from build123d import *

# Parameters (mm, degrees)
BOSS_EXTRUDE4_DEPTH = 107
BOSS_EXTRUDE5_DEPTH = 2.31
SKETCH7_W           = 102.38
SKETCH7_H           = 83.08
CUT_EXTRUDE4_DEPTH  = 2.31
BOSS_EXTRUDE6_DEPTH = 2.31
CUT_EXTRUDE6_DEPTH  = 2.31
CUT_EXTRUDE7_DEPTH  = 70
SKETCH12_W          = 91.85
SKETCH12_H          = 11.6
CUT_EXTRUDE8_DEPTH  = 90


with BuildPart() as part:
    # Sketch1 → Boss-Extrude4 (new body)
    with BuildSketch(Plane(origin=(0, 0, 0), x_dir=(0, 0, -1), z_dir=(1, 0, 0))):
        with BuildLine():
            Line((0, 0), (87.7, 0))
            Line((87.7, 0), (87.7, 14.19))
            ThreePointArc((87.7, 14.19), (87.023416665, 15.823416665), (85.39, 16.5))
            Line((85.39, 16.5), (76.167, 16.5))
            ThreePointArc((76.167, 16.5), (74.533583335, 17.176583335), (73.857, 18.81))
            Line((73.857, 18.81), (73.857, 34.19))
            ThreePointArc((73.857, 34.19), (73.180416665, 35.823416665), (71.547, 36.5))
            Line((71.547, 36.5), (69.1628, 36.5))
            ThreePointArc((69.1628, 36.5), (67.529383335, 37.176583335), (66.8528, 38.81))
            Line((66.8528, 38.81), (66.8528, 45.417647019))
            ThreePointArc((66.8528, 45.417647019), (43.8531, 48.5), (20.8534, 45.417647019))
            Line((20.8534, 45.417647019), (20.8534, 38.81))
            ThreePointArc((20.8534, 38.81), (20.176816665, 37.176583335), (18.5434, 36.5))
            Line((18.5434, 36.5), (16.153, 36.5))
            ThreePointArc((16.153, 36.5), (14.519583335, 35.823416665), (13.843, 34.19))
            Line((13.843, 34.19), (13.843, 18.81))
            ThreePointArc((13.843, 18.81), (13.166416665, 17.176583335), (11.533, 16.5))
            Line((11.533, 16.5), (2.31, 16.5))
            ThreePointArc((2.31, 16.5), (0.676583335, 15.823416665), (0, 14.19))
            Line((0, 14.19), (0, 0))
        make_face()
        with BuildLine():
            Line((16.153, 34.19), (16.153, 18.81))
            ThreePointArc((16.153, 18.81), (14.799833329, 15.543166671), (11.533, 14.19))
            Line((11.533, 14.19), (2.31, 14.19))
            Line((2.31, 14.19), (2.31, 2.31))
            Line((2.31, 2.31), (85.39, 2.31))
            Line((85.39, 2.31), (85.39, 14.19))
            Line((85.39, 14.19), (76.167, 14.19))
            ThreePointArc((76.167, 14.19), (72.900166671, 15.543166671), (71.547, 18.81))
            Line((71.547, 18.81), (71.547, 34.19))
            Line((71.547, 34.19), (69.1628, 34.19))
            ThreePointArc((69.1628, 34.19), (65.895966671, 35.543166671), (64.5428, 38.81))
            Line((64.5428, 38.81), (64.5428, 43.634774003))
            ThreePointArc((64.5428, 43.634774003), (43.8531, 46.19), (23.1634, 43.634774003))
            Line((23.1634, 43.634774003), (23.1634, 38.81))
            ThreePointArc((23.1634, 38.81), (21.810233329, 35.543166671), (18.5434, 34.19))
            Line((18.5434, 34.19), (16.153, 34.19))
        make_face(mode=Mode.SUBTRACT)
    extrude(amount=BOSS_EXTRUDE4_DEPTH)

    # Sketch6 → Boss-Extrude5 (add)
    with BuildSketch(Plane.ZY):
        with BuildLine():
            Line((-85.39, 14.19), (-85.39, 2.31))
            Line((-85.39, 2.31), (-2.31, 2.31))
            Line((-2.31, 2.31), (-2.31, 14.19))
            Line((-2.31, 14.19), (-11.533, 14.19))
            ThreePointArc((-11.533, 14.19), (-14.799833329, 15.543166671), (-16.153, 18.81))
            Line((-16.153, 18.81), (-16.153, 34.19))
            Line((-16.153, 34.19), (-18.5434, 34.19))
            ThreePointArc((-18.5434, 34.19), (-21.810233329, 35.543166671), (-23.1634, 38.81))
            Line((-23.1634, 38.81), (-23.1634, 43.634774003))
            ThreePointArc((-23.1634, 43.634774003), (-43.8531, 46.19), (-64.5428, 43.634774003))
            Line((-64.5428, 43.634774003), (-64.5428, 38.81))
            ThreePointArc((-64.5428, 38.81), (-65.895966671, 35.543166671), (-69.1628, 34.19))
            ThreePointArc((-69.1628, 34.19), (-69.258906021, 34.189020865), (-69.355012042, 34.19))
            Line((-69.355012042, 34.19), (-71.547, 34.19))
            Line((-71.547, 34.19), (-71.547, 18.81))
            ThreePointArc((-71.547, 18.81), (-72.900166671, 15.543166671), (-76.167, 14.19))
            Line((-76.167, 14.19), (-85.39, 14.19))
        make_face()
    extrude(amount=-BOSS_EXTRUDE5_DEPTH)

    # Sketch7 → Cut-Extrude4 (cut)
    with BuildSketch(Plane.XZ):
        with Locations((53.5, -43.85)):
            Rectangle(SKETCH7_W, SKETCH7_H)
    extrude(amount=-CUT_EXTRUDE4_DEPTH, mode=Mode.SUBTRACT)

    # Sketch8 → Boss-Extrude6 (add)
    with BuildSketch(Plane(origin=(107, 0, 0), x_dir=(0, 0, -1), z_dir=(1, 0, 0))):
        with BuildLine():
            Line((2.31, 14.19), (2.31, 2.31))
            Line((2.31, 2.31), (85.39, 2.31))
            Line((85.39, 2.31), (85.39, 14.19))
            Line((85.39, 14.19), (76.167, 14.19))
            ThreePointArc((76.167, 14.19), (72.900166671, 15.543166671), (71.547, 18.81))
            Line((71.547, 18.81), (71.547, 34.19))
            Line((71.547, 34.19), (69.355012042, 34.19))
            ThreePointArc((69.355012042, 34.19), (69.258906021, 34.189020865), (69.1628, 34.19))
            ThreePointArc((69.1628, 34.19), (65.895966671, 35.543166671), (64.5428, 38.81))
            Line((64.5428, 38.81), (64.5428, 43.634774003))
            ThreePointArc((64.5428, 43.634774003), (43.8531, 46.19), (23.1634, 43.634774003))
            Line((23.1634, 43.634774003), (23.1634, 38.81))
            ThreePointArc((23.1634, 38.81), (21.810233329, 35.543166671), (18.5434, 34.19))
            Line((18.5434, 34.19), (16.153, 34.19))
            Line((16.153, 34.19), (16.153, 18.81))
            ThreePointArc((16.153, 18.81), (14.799833329, 15.543166671), (11.533, 14.19))
            Line((11.533, 14.19), (2.31, 14.19))
        make_face()
    extrude(amount=-BOSS_EXTRUDE6_DEPTH)

    # Sketch9 → Cut-Extrude6 (cut)
    with BuildSketch(Plane(origin=(0, 16.5, 0), x_dir=(1, 0, 0), z_dir=(0, 1, 0))):
        with BuildLine():
            Line((25, 83.7785), (82, 83.7785))
            ThreePointArc((82, 83.7785), (85, 80.7785), (82, 77.7785))
            Line((82, 77.7785), (25, 77.7785))
            ThreePointArc((25, 77.7785), (22, 80.7785), (25, 83.7785))
        make_face()
        with BuildLine():
            Line((25, 9.9215), (82, 9.9215))
            ThreePointArc((82, 9.9215), (85, 6.9215), (82, 3.9215))
            Line((82, 3.9215), (25, 3.9215))
            ThreePointArc((25, 3.9215), (22, 6.9215), (25, 9.9215))
        make_face()
    extrude(amount=-CUT_EXTRUDE6_DEPTH, mode=Mode.SUBTRACT)

    # Sketch11 → Cut-Extrude7 (cut)
    with BuildSketch(Plane.XY.offset(-13.843)):
        with BuildLine():
            Line((28.648320597, 30.5), (28.648320597, 22.5))
            ThreePointArc((28.648320597, 22.5), (29.898320597, 21.25), (31.148320597, 22.5))
            Line((31.148320597, 22.5), (31.148320597, 30.5))
            ThreePointArc((31.148320597, 30.5), (29.898320597, 31.75), (28.648320597, 30.5))
        make_face()
        with BuildLine():
            Line((38.648320597, 30.5), (38.648320597, 22.5))
            ThreePointArc((38.648320597, 22.5), (39.898320597, 21.25), (41.148320597, 22.5))
            Line((41.148320597, 22.5), (41.148320597, 30.5))
            ThreePointArc((41.148320597, 30.5), (39.898320597, 31.75), (38.648320597, 30.5))
        make_face()
        with BuildLine():
            Line((43.648320597, 30.5), (43.648320597, 22.5))
            ThreePointArc((43.648320597, 22.5), (44.898320597, 21.25), (46.148320597, 22.5))
            Line((46.148320597, 22.5), (46.148320597, 30.5))
            ThreePointArc((46.148320597, 30.5), (44.898320597, 31.75), (43.648320597, 30.5))
        make_face()
        with BuildLine():
            Line((48.648320597, 30.5), (48.648320597, 22.5))
            ThreePointArc((48.648320597, 22.5), (49.898320597, 21.25), (51.148320597, 22.5))
            Line((51.148320597, 22.5), (51.148320597, 30.5))
            ThreePointArc((51.148320597, 30.5), (49.898320597, 31.75), (48.648320597, 30.5))
        make_face()
        with BuildLine():
            Line((58.648320597, 30.5), (58.648320597, 22.5))
            ThreePointArc((58.648320597, 22.5), (59.898320597, 21.25), (61.148320597, 22.5))
            Line((61.148320597, 22.5), (61.148320597, 30.5))
            ThreePointArc((61.148320597, 30.5), (59.898320597, 31.75), (58.648320597, 30.5))
        make_face()
        with BuildLine():
            Line((63.648320597, 30.5), (63.648320597, 22.5))
            ThreePointArc((63.648320597, 22.5), (64.898320597, 21.25), (66.148320597, 22.5))
            Line((66.148320597, 22.5), (66.148320597, 30.5))
            ThreePointArc((66.148320597, 30.5), (64.898320597, 31.75), (63.648320597, 30.5))
        make_face()
        with BuildLine():
            Line((33.648320597, 30.5), (33.648320597, 22.5))
            ThreePointArc((33.648320597, 22.5), (34.898320597, 21.25), (36.148320597, 22.5))
            Line((36.148320597, 22.5), (36.148320597, 30.5))
            ThreePointArc((36.148320597, 30.5), (34.898320597, 31.75), (33.648320597, 30.5))
        make_face()
        with BuildLine():
            Line((53.648320597, 30.5), (53.648320597, 22.5))
            ThreePointArc((53.648320597, 22.5), (54.898320597, 21.25), (56.148320597, 22.5))
            Line((56.148320597, 22.5), (56.148320597, 30.5))
            ThreePointArc((56.148320597, 30.5), (54.898320597, 31.75), (53.648320597, 30.5))
        make_face()
        with BuildLine():
            Line((68.648320597, 30.5), (68.648320597, 22.5))
            ThreePointArc((68.648320597, 22.5), (69.898320597, 21.25), (71.148320597, 22.5))
            Line((71.148320597, 22.5), (71.148320597, 30.5))
            ThreePointArc((71.148320597, 30.5), (69.898320597, 31.75), (68.648320597, 30.5))
        make_face()
        with BuildLine():
            Line((76.148320597, 30.5), (76.148320597, 22.5))
            ThreePointArc((76.148320597, 22.5), (74.898320597, 21.25), (73.648320597, 22.5))
            Line((73.648320597, 22.5), (73.648320597, 30.5))
            ThreePointArc((73.648320597, 30.5), (74.898320597, 31.75), (76.148320597, 30.5))
        make_face()
        with BuildLine():
            Line((78.648320597, 30.5), (78.648320597, 22.5))
            ThreePointArc((78.648320597, 22.5), (79.898320597, 21.25), (81.148320597, 22.5))
            Line((81.148320597, 22.5), (81.148320597, 30.5))
            ThreePointArc((81.148320597, 30.5), (79.898320597, 31.75), (78.648320597, 30.5))
        make_face()
    extrude(amount=-CUT_EXTRUDE7_DEPTH, mode=Mode.SUBTRACT)

    # Sketch12 → Cut-Extrude8 (cut)
    with BuildSketch(Plane.XY):
        with Locations((53.505, 5.8)):
            Rectangle(SKETCH12_W, SKETCH12_H)
    extrude(amount=-CUT_EXTRUDE8_DEPTH, mode=Mode.SUBTRACT)


solid = part.part
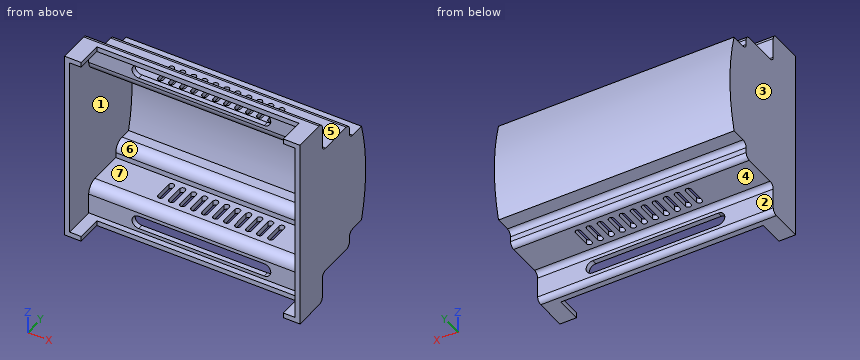
Can you work these out from the model? Positions are in its coordinate system, mm. Face numbers are marked on the shaded views. A direction names the side the tool comes from. Coordinates: 2 decimals unless noted, no trailing zeros. Loops run counter-clockwise (first coordinate to the right, second up) from the corner with the lowest first, then second, coordinate; pieces in that order, holes last. Notation, with made-up numbers: M 19.25,-28.5 L 28.25,-28.5 A17 cw 28.25,4.5 Z; hole C 89.25,-12.5 d8. An arc over 180 degrees is marked long. Return JSON: item names as keys, results as strings. Group by question number.
Item 1: Thinking about a two-plate mould opening in Z: for the marked faces 4, 5, 6 and 7, which applies, released by +Z, released by -Z, zero draft, split by the parting line, or undercut?
Item 2: Imagine slicing it at C-C (z = -29.5). Please give me the cut outline in (x, y).
Item 3: Imagine slicing it at B-B (z = -45.5). Please give me the cut outline in (x, y).
Item 4: Imagine slicing it at A-A (y = 28.5). Give the number of separate pieces and of enclosed holes in the cut face, and give its area (3 significant figures).
Item 5: On a 3-axis mill with a long thin cutter (end or side, diameter ignored), from which of +Z, -Z, +X, -X, +Y, -Y can I reach the whole of each face in a straight line? I mean the marked faces 1, 2 and 3. Say none if no direction works.
Item 6: If I drill on L1, parallel to Z at x = 6.5, y = 39; L2, parallel to Z at x = 66.5, y = 26.5; L3, parallel to X at y = 36, z = -46, over which ranges is the centre line in solid material (lowest first)? Write a range as from..to.
Item 7: I'm going to push flat-ended pins straight in: pin 1 Ø3 at (x, z) = (26.5, -9.5) entering from +Y; pin 2 Ø1.2 at (x, y) = (61.5, 15) entering from +Z; pin 3 Ø1.2 at (x, z) = (40.5, -86.5) entering from -Y. Where does each tip first touch, or does it pass through?
Verdict:
{
 "1": {"face 4": "released by -Z", "face 5": "released by +Z", "face 6": "undercut", "face 7": "undercut"},
 "2": {"outline": "M 0,0 L 2.31,0 L 2.31,44.97 L 104.69,44.97 L 104.69,0 L 107,0 L 107,47.31 L 0,47.31 Z"},
 "3": {"outline": "M 0,0 L 2.31,0 L 2.31,46.17 L 104.69,46.17 L 104.69,0 L 107,0 L 107,48.48 L 0,48.48 Z"},
 "4": {"separate pieces": "22", "enclosed holes": "0", "area": "623 mm^2"},
 "5": {"face 1": "-Y", "face 2": "-Z, +X, -X, +Y", "face 3": "+Z, -Z, -X, +Y, -Y"},
 "6": {"L1": "z = -66.85..-64.54, -23.16..-20.85", "L2": "z = -73.86..-71.55, -16.15..-13.84", "L3": "x = 0..2.31, 104.69..107"},
 "7": {"pin 1": "stops at y = 16.5", "pin 2": "stops at z = -0.01", "pin 3": "stops at y = 11.6"}
}
